The figure shows three views and two pictorial views of one solid part (mm, origin at its lowest corner). Answer the questions. A direction names the side the tool comes from. Round coordinates to 2 decimals unless told otherwise and drop trailing zeros. Order: outer loops, then holes, each group sorted by start corner. A loop starts at its lowest first (then second) coordinate and runs counter-clockwise, first axis right, second up. Notation, with made-up numbers: (-6.75, 68.5) -> (8.25, 68.5) arc R17 ccw to (8.25, 73.5) -> close; hole circle Ø9 at (-34.5, 49). An arc over 180 degrees is marked (long way). Answer as a JSON object with one key per item and string values. Group by question number.
Item 1: Section C-C, the plane z = 14.75 is taken. Write down the section's boundary in (x, y), plus the area to 3 significant figures.
Item 2: Section D-D, the plane y = 4 is taken. Write down the section's boundary in (x, z).
Item 3: Given P1, Ø1, axis at y = 7, z = 6, coming from the +X side; P2, Ø0.8, axis at x = 3.5, y = 7.5, coming from the +Z side; P3, Ø1, axis at x = 7, z = 24, coming from the -Y side, each flat-ended and moving along its own axis, determine where each tip first touches the part or whether it passes through.
Item 4: Section A-A, the plane x = 4 is taken. Write down the section's boundary in (y, z).
Item 5: For the marked faces 1, 2 and 3, determine the directions among +Z, -Z, +X, -X, +Y, -Y from which every point of the face is accessible in a straight line to the end or side of a thin tool.
Item 6: Section B-B, the plane y = 6.25 is taken. Write down the section's boundary in (x, z), plus the area to 3 significant figures.
Item 7: Consider probe 1 along Y at (x, z) = (4, 5); probe 2 along Z at (x, y) = (5, 7.75); probe 3 along Z at (x, y) = (2.25, 0.75). Determine where each line is inside the solid, lowest interval first. Write a range as from..to.
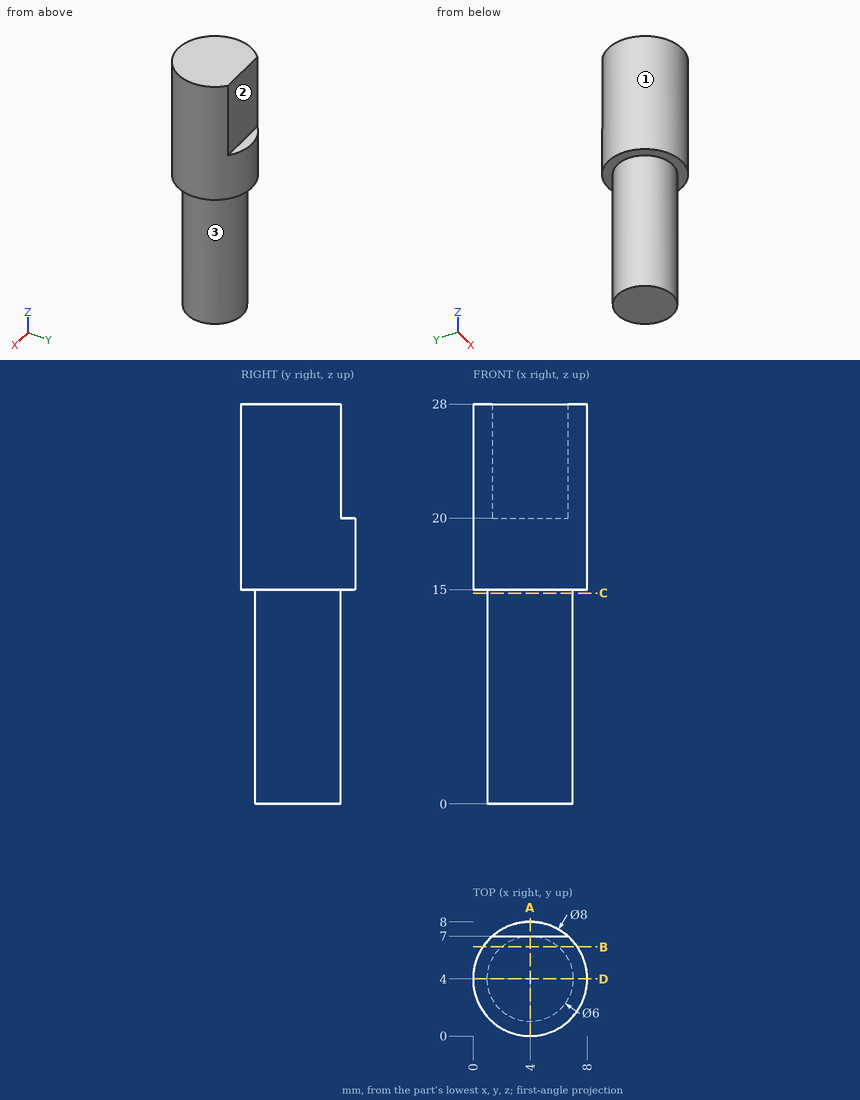
Values found:
{
 "1": {"outline": "circle Ø6 at (4, 4)", "area": "28.3 mm2"},
 "2": {"outline": "(0, 15) -> (1, 15) -> (1, 0) -> (7, 0) -> (7, 15) -> (8, 15) -> (8, 28) -> (0, 28) -> close"},
 "3": {"P1": "x = 5.66", "P2": "z = 20", "P3": "y = 0.88"},
 "4": {"outline": "(0, 15) -> (1, 15) -> (1, 0) -> (7, 0) -> (7, 15) -> (8, 15) -> (8, 20) -> (7, 20) -> (7, 28) -> (0, 28) -> close"},
 "5": {"face 1": "+Z, -Z", "face 2": "+Z, +X, -X, +Y", "face 3": "-Z"},
 "6": {"outline": "(0.69, 15) -> (2.02, 15) -> (2.02, 0) -> (5.98, 0) -> (5.98, 15) -> (7.31, 15) -> (7.31, 28) -> (0.69, 28) -> close", "area": "146 mm2"},
 "7": {"probe 1": "1..7", "probe 2": "15..20", "probe 3": "15..28"}
}
